Check sheet for the modelled part. Datum: model origin and axes. Units: mm. A direction names the side the tool comes from. Give positions to 0.01 mm unless a question says otherwise; leave off trailing zeros. Write each loop counter-clockwise with the first axis right and the second up, starting at its lowest first coordinate (ties: lowest second). Pieces come first, ordered by that corner, then holes. Notation, with made-up numbers: (59, 26.25) -> (92, 26.25) arc R16 cw to (92, 55.25) -> close; hole circle Ø6 at (-6.75, -30.75). An arc over 180 degrees is marked (long way). Use a Markdown table: item, result. Add a question column.
1. Scan lines: probe 1 along X at (y, z) = (-15.5, 5); probe 2 along Z at (x, y) = (-26, 5.5); probe 3 along X at (y, z) = (-22.5, 121.5). Record each from-to range of solid material in increasing order. Write a range as [from, to].
2. Release check for a two-part mould opening along X. For faces 4 (the cylindrical face through (42.169, -23.373, 4.504)), 5 (the flat face through (-153.405, -13, 2)), 6 (the flat face through (-55, -13, 3)), 7 (the flat face through (-152, -3.513, 4)) record: released by +X, released by -X, zero draft, split by the parting line, or undercut.
3. Cross-section at C-C (x = -85.5). Enter the section's corners in (y, z), then the cut area to 3 significant figures.
4. Set-up check for faces 1 (the flat face through (41, -23.513, 162)), 2 (the flat face through (-152, -23.513, 4)), 3 (the flat face through (45, -13.513, 83)): record each of +Z, -Z, +X, -X, +Y, -Y from which the full face is reachable in a straight line by a thin tool's end or side.
5. Gauge pin test, flat ends, axial feed: P1, Ø1.8, axis at x = -151.41, z = 5, coming from the +Y side; P2, Ø9, axis at x = 41, z = 109, coming from the +Y side; P3, Ø2, axis at x = -90, y = -6.5, coming from the +Z side; P4, Ø1.2, axis at x = -152, z = 5, coming from the -Y side. Record the tip position at first contact, or that the pin passes through.
6. Cross-section at B-B (z = 61). Enter the section's corners in (x, y).
7. Cross-section at A-A (y = -29). Enter the section's corners in (x, z).
from build123d import *

# Parameters (mm, degrees)
SKETCH1_W           = 200
SKETCH1_H           = 40
BOSS_EXTRUDE1_DEPTH = 3
SKETCH2_W           = 160
SKETCH2_H           = 20
BOSS_EXTRUDE2_DEPTH = 3
FILLET1_R           = 5
SKETCH3_R           = 1
BOSS_EXTRUDE3_DEPTH = 10
LPATTERN1_COUNT     = 2
LPATTERN1_PITCH     = 20
SKETCH4_R           = 1
BOSS_EXTRUDE4_DEPTH = 10


with BuildPart() as part:
    # Sketch1 → Boss-Extrude1 (new body)
    with BuildSketch(Plane.XY):
        with Locations((-53.405017921, -13.512544803)):
            Rectangle(SKETCH1_W, SKETCH1_H)
    extrude(amount=BOSS_EXTRUDE1_DEPTH)

    # Sketch2 → Boss-Extrude2 (add)
    with BuildSketch(Plane(origin=(46.594982079, 0, 0), x_dir=(0, 0, -1), z_dir=(1, 0, 0))):
        with Locations((-83, -23.512544803)):
            Rectangle(SKETCH2_W, SKETCH2_H)
    extrude(amount=-BOSS_EXTRUDE2_DEPTH)

    # Fillet1
    fillet1_edges = [part.edges().sort_by_distance(p)[0] for p in [
        (43.594982079, -23.512544803, 3),
    ]]
    fillet(fillet1_edges, radius=FILLET1_R)

    # Sketch3 → Boss-Extrude3 (add)
    with BuildSketch(Plane(origin=(0, 6.487455197, 0), x_dir=(1, 0, 0), z_dir=(0, 1, 0))):
        with BuildLine():
            Line((-153.405017921, -3), (-153.405017921, -5))
            ThreePointArc((-153.405017921, -5), (-149.990804359, -6.414213562), (-151.405017921, -3))
            Line((-151.405017921, -3), (-153.405017921, -3))
        make_face()
        with Locations(Location((-151.405017921, -5, 0), (0, 0, 270))):
            Circle(SKETCH3_R, mode=Mode.SUBTRACT)
    boss_extrude3 = extrude(amount=-BOSS_EXTRUDE3_DEPTH)

    # LPattern1: Boss-Extrude3 ×2
    with Locations(*[(0, -i * LPATTERN1_PITCH, 0) for i in range(1, LPATTERN1_COUNT)]):
        add(boss_extrude3)

    # Sketch4 → Boss-Extrude4 (add)
    with BuildSketch(Plane.XZ.offset(33.512544803)):
        with BuildLine():
            Line((43.594982079, 163), (41.594982079, 163))
            ThreePointArc((41.594982079, 163), (40.180768516, 159.585786438), (43.594982079, 161))
            Line((43.594982079, 161), (43.594982079, 163))
        make_face()
        with Locations(Location((41.594982079, 161, 0), (0, 0, 270))):
            Circle(SKETCH4_R, mode=Mode.SUBTRACT)
    extrude(amount=-BOSS_EXTRUDE4_DEPTH)


solid = part.part
Worked answers:
| question | item | result |
|---|---|---|
| 1 | probe 1 | x = [-153.41, -152.41], [-150.41, -149.41], [42.59, 46.59] |
| 1 | probe 2 | z = [0, 3] |
| 1 | probe 3 | x = [43.59, 46.59] |
| 2 | face 4 | undercut |
| 2 | face 5 | released by -X |
| 2 | face 6 | undercut |
| 2 | face 7 | zero draft |
| 3 | outline | (-33.51, 0) -> (6.49, 0) -> (6.49, 3) -> (-33.51, 3) -> close |
| 3 | area | 120 mm² |
| 4 | face 1 | +Z, -X, +Y |
| 4 | face 2 | +Z, -X, -Y |
| 4 | face 3 | +Z, +X, -X, +Y |
| 5 | P1 | passes through |
| 5 | P2 | stops at y = -13.51 |
| 5 | P3 | stops at z = 3 |
| 5 | P4 | stops at y = -23.51 |
| 6 | outline | (43.59, -33.51) -> (46.59, -33.51) -> (46.59, -13.51) -> (43.59, -13.51) -> close |
| 7 | outline | (-153.41, 0) -> (46.59, 0) -> (46.59, 163) -> (41.59, 163) arc R2 ccw (long way) to (43.59, 161) -> (43.59, 8) arc R5 cw to (38.59, 3) -> (-153.41, 3) -> close; hole circle Ø2 at (41.59, 161) |
